from build123d import *

# Parameters (mm, degrees)
F0_W     = 152.4
F0_H     = 109.22
F1_DEPTH = 152.4
F2_T     = -3.175
F3_W     = 101.6
F3_H     = 45.72
F4_DEPTH = 152.401
F5_W     = 146.05
F5_H     = 22.225
F5_H_2   = 123.825
F6_DEPTH = 25.4
F8_DEPTH = 152.401
F9_R     = 2.54
F10_R    = 5.08


with BuildPart() as f1:
    # F0 (on Front) → F1 (new body)
    with BuildSketch(Plane.XZ):
        with Locations((76.2, 54.61)):
            Rectangle(F0_W, F0_H)
    extrude(amount=F1_DEPTH)

    # F2
    f2_openings = [f1.faces().sort_by_distance(p)[0] for p in [
        (76.2, -152.4, 54.61),
    ]]
    offset(amount=F2_T, openings=f2_openings)

    # F3 (on face) → F4 (cut, through all)
    with BuildSketch(Plane.YZ.offset(152.4)):
        with Locations((-76.2, 86.36)):
            Rectangle(F3_W, F3_H)
    extrude(amount=-F4_DEPTH, mode=Mode.SUBTRACT)

    # F5 (on face) → F6 (cut)
    with BuildSketch(Plane.XY.offset(109.22)):
        with Locations((76.2, -138.1125)):
            Rectangle(F5_W, F5_H)
        with Locations((76.2, -65.0875)):
            Rectangle(F5_W, F5_H_2)
    extrude(amount=-F6_DEPTH, mode=Mode.SUBTRACT)

    # F7 (on face) → F8 (cut, through all)
    with BuildSketch(Plane.YZ.offset(152.4)):
        Polygon((-31.75, 0), (0, 0), (0, 31.75), align=None)
    extrude(amount=-F8_DEPTH, mode=Mode.SUBTRACT)

    # F9
    f9_edges = [f1.edges().sort_by_distance(p)[0] for p in [
        (3.175, -90.4875, 3.175),
        (3.175, -3.175, 68.8975),
        (149.225, -3.175, 68.8975),
        (1.5875, -25.4, 63.5),
        (150.8125, -25.4, 63.5),
        (150.8125, -127, 63.5),
        (1.5875, -127, 63.5),
        (149.225, -90.4875, 3.175),
    ]]
    fillet(f9_edges, radius=F9_R)

    # F10
    f10_edges = [f1.edges().sort_by_distance(p)[0] for p in [
        (3.175, -149.225, 107.6325),
        (149.225, -149.225, 107.6325),
    ]]
    fillet(f10_edges, radius=F10_R)


solid = f1.part
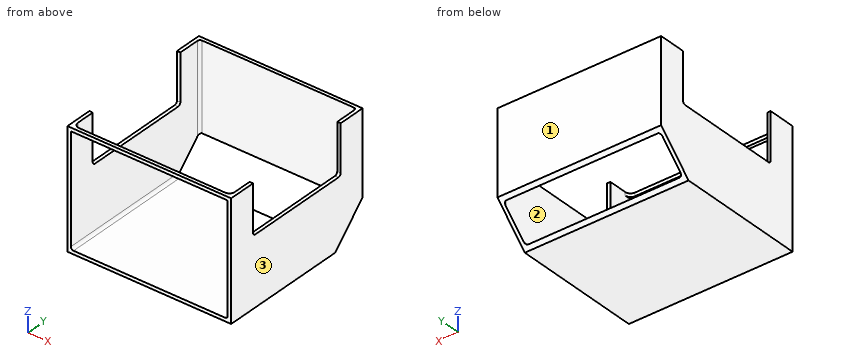
Here's how the part is built. I have some questions about the finished solid (model axes, mm). Face numbers are marked on the shaded views. Coordinates: 2 decimals unless noted, no trailing zeros. Write each loop counter-clockwise with the first axis right and the second up, starting at its lowest first coordinate (ties: lowest second). Pieces come first, ordered by that corner, then holes.
Item 1: I want a section at D-D on y = -39.5. Write out the boundary of the cut face in (x, z) (3 decimals).
Item 2: I want a section at B-B on z = 12.5. Write out the boundary of the cut face in (x, y) (3 decimals), and give its area (4 significant figures).
Item 3: If we mould it in two halves opening along X, with no side actions, what happens to the marked faces 1, 2 and 3? For each: +X half, -X half, draft (parallel to the pull), parting line (faces both ways), or undercut.
Item 4: If I drill on line 1 (X direction, y = -15, z = 86) (3 decimals); line 2 (Y direction, x = 27, z = 60) (3 decimals); line 3 (Z direction, x = 49.5, y = -128) (3 decimals), over which ranges is the centre line in solid material (lowest first)?
Item 5: I want a section at A-A on z = 94.5. Write out the boundary of the cut face in (x, y) (3 decimals).
Item 6: Will these pins go through, and if not, where does the flat tip stop? pin 1 (1.6 mm diameter, centred on x = 150.5, y = -58.5, fed in from +Z); pin 2 (6 mm diameter, centred on x = 126, z = 56, fed in from +Y); pin 3 (1.5 mm diameter, centred on x = 19, z = 35.5, fed in from -Y) (3 decimals).
Item 7: I want a section at C-C on x = 36. Write out the boundary of the cut face in (y, z) (3 decimals), and give its area (3 significant figures).
Findings below:
1. outline: (0, 0) - (152.4, 0) - (152.4, 63.5) - (149.225, 63.5) - (149.225, 5.715) arc R2.54 cw to (146.685, 3.175) - (5.715, 3.175) arc R2.54 cw to (3.175, 5.715) - (3.175, 63.5) - (0, 63.5) - close
2. outline: (0, -152.4) - (3.175, -152.4) - (3.175, -19.25) - (0, -19.25) - close; (149.225, -152.4) - (152.4, -152.4) - (152.4, -19.25) - (149.225, -19.25) - close
2. area: 845.5 mm2
3. face 1: draft
3. face 2: undercut
3. face 3: +X half
4. line 1: x = 0 to 3.175, 149.225 to 152.4
4. line 2: y = -3.175 to 0
4. line 3: z = 0 to 3.175
5. outline: (0, -152.4) - (3.175, -152.4) - (3.175, -127) - (0, -127) - close; (0, -25.4) - (3.175, -25.4) - (3.175, -5.715) arc R2.54 cw to (5.715, -3.175) - (146.685, -3.175) arc R2.54 cw to (149.225, -5.715) - (149.225, -25.4) - (152.4, -25.4) - (152.4, 0) - (0, 0) - close; (149.225, -152.4) - (152.4, -152.4) - (152.4, -127) - (149.225, -127) - close
6. pin 1: stops at z = 63.5
6. pin 2: stops at y = 0
6. pin 3: stops at y = -3.175
7. outline: (-152.4, 0) - (-31.75, 0) - (-28.575, 3.175) - (-152.4, 3.175) - close; (-152.4, 106.045) - (-149.225, 106.045) - (-149.225, 109.22) - (-152.4, 109.22) - close; (-3.175, 28.575) - (0, 31.75) - (0, 109.22) - (-3.175, 109.22) - close
7. area: 649 mm2
